Read the model definition and answer for the solid it produces. Units are mm, in the model's axes. Face numbers are marked on the shaded views. A direction names the side the tool comes from. Give positions to 0.01 mm unless a question says otherwise; leave off trailing zeros. Order: outer loops, then holes, each group sorted by start corner. A loop starts at its lowest first (then second) coordinate and runs counter-clockwise, first axis right, second up.
Item 1: Which of the six approach directions +Z, -Z, +X, -X, +Y, -Y give full straight-line access (tool end or side, diameter ignored) to the marked faces 1 and 2?
Item 2: A cutting plane is placed at C-C (z = 7.25). Write down the section's boundary in (x, y).
Item 3: A cutting plane is placed at D-D (x = 12). Write down the section's boundary in (y, z), plus the area to 3 significant figures.
Item 4: Find the intervals of material crossed by line 1 along Y through (x, z) = (60, 5.75); line 2 along Y through (x, z) = (41.5, 3); line 3 along X through (y, z) = (19, 4), in increasing order.
Item 5: A cutting plane is placed at A-A (z = 1.75). Write down the section's boundary in (x, y), plus the area to 3 significant figures.
Item 6: A cutting plane is placed at B-B (y = 30.5). Write down the section's boundary in (x, z).
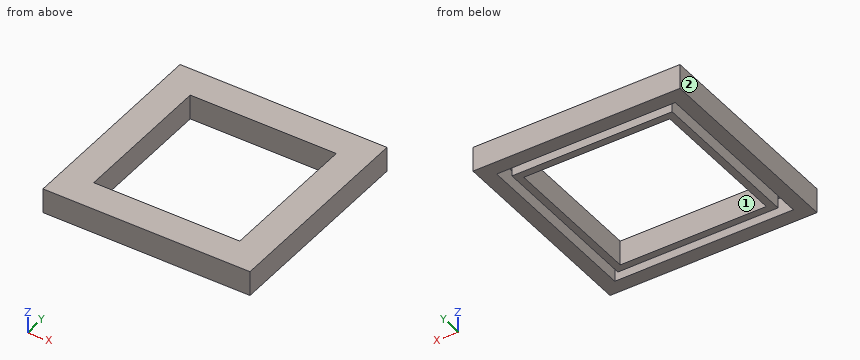
from build123d import *

# Parameters (mm, degrees)
SKETCH1_W             = 57.404
SKETCH1_H             = 57.15
SKETCH1_W_2           = 52.324
SKETCH1_H_2           = 52.07
BOSS_EXTRUDE1_DEPTH   = 6.35
SKETCH1_W_3           = 74.168
SKETCH1_H_3           = 73.914
BOSS_EXTRUDE1_2_DEPTH = 6.35
SKETCH2_W             = 74.168
SKETCH2_H             = 73.914
SKETCH2_W_2           = 52.324
SKETCH2_H_2           = 52.07
BOSS_EXTRUDE2_DEPTH   = 2.54


with BuildPart() as part:
    # Sketch1 → Boss-Extrude1 (new body)
    with BuildSketch(Plane.XY):
        with Locations((32.004, 31.877)):
            Rectangle(SKETCH1_W, SKETCH1_H)
        with Locations((32.004, 31.877)):
            Rectangle(SKETCH1_W_2, SKETCH1_H_2, mode=Mode.SUBTRACT)
    extrude(amount=BOSS_EXTRUDE1_DEPTH)



with BuildPart() as body_2:
    # Sketch1 → Boss-Extrude1 2 (new body)
    with BuildSketch(Plane.XY):
        with Locations((32.004, 31.877)):
            Rectangle(SKETCH1_W_3, SKETCH1_H_3)
        Polygon((0, 0), (64.008, 0), (64.008, 63.754), (60.706, 63.754), (3.302, 63.754), (0, 63.754), align=None, mode=Mode.SUBTRACT)
    extrude(amount=BOSS_EXTRUDE1_2_DEPTH)


with BuildPart() as part_1:
    add(part.part)

    add(body_2.part)  # Boss-Extrude2 merges body 2
    # Sketch2 → Boss-Extrude2 (add)
    with BuildSketch(Plane.XY.offset(6.35)):
        with Locations((32.004, 31.877)):
            Rectangle(SKETCH2_W, SKETCH2_H)
        with Locations((32.004, 31.877)):
            Rectangle(SKETCH2_W_2, SKETCH2_H_2, mode=Mode.SUBTRACT)
    extrude(amount=BOSS_EXTRUDE2_DEPTH)


solid = part_1.part
Response values:
1. face 1: +Z, -Z
1. face 2: +Z, -Z, -X, +Y, -Y
2. outline: (-5.08, -5.08) - (69.09, -5.08) - (69.09, 68.83) - (-5.08, 68.83) - close; hole (5.84, 5.84) - (58.17, 5.84) - (58.17, 57.91) - (5.84, 57.91) - close
3. outline: (-5.08, 0) - (0, 0) - (0, 6.35) - (3.3, 6.35) - (3.3, 0) - (5.84, 0) - (5.84, 8.89) - (-5.08, 8.89) - close; (57.91, 0) - (60.45, 0) - (60.45, 6.35) - (63.75, 6.35) - (63.75, 0) - (68.83, 0) - (68.83, 8.89) - (57.91, 8.89) - close
3. area: 152 mm2
4. line 1: y = -5.08 to 0, 3.3 to 60.45, 63.75 to 68.83
4. line 2: y = -5.08 to 0, 3.3 to 5.84, 57.91 to 60.45, 63.75 to 68.83
4. line 3: x = -5.08 to 0, 3.3 to 5.84, 58.17 to 60.71, 64.01 to 69.09
5. outline: (-5.08, -5.08) - (69.09, -5.08) - (69.09, 68.83) - (-5.08, 68.83) - close; (3.3, 3.3) - (60.71, 3.3) - (60.71, 60.45) - (3.3, 60.45) - close; hole (0, 0) - (64.01, 0) - (64.01, 63.75) - (0, 63.75) - close; hole (5.84, 5.84) - (58.17, 5.84) - (58.17, 57.91) - (5.84, 57.91) - close
5. area: 1,960 mm2
6. outline: (-5.08, 0) - (0, 0) - (0, 6.35) - (3.3, 6.35) - (3.3, 0) - (5.84, 0) - (5.84, 8.89) - (-5.08, 8.89) - close; (58.17, 0) - (60.71, 0) - (60.71, 6.35) - (64.01, 6.35) - (64.01, 0) - (69.09, 0) - (69.09, 8.89) - (58.17, 8.89) - close
